```python
from build123d import *

# Parameters (mm, degrees)
SKETCH2_R                      = 2
BOSS_EXTRUDE1_DEPTH            = 10
CUT_EXTRUDE2_DEPTH             = 31.479501308
CUT_EXTRUDE2_DEPTH_BACK        = 31.479501308
SKETCH4_W                      = 15
SKETCH4_H                      = 9.2
CUT_EXTRUDE1_REACH             = 37.057
SKETCH3_R                      = 4.5
FILLET3_R                      = 1.5
FILLET4_R                      = 2
CUT_EXTRUDE3_REACH             = 31.082
SKETCH5_R                      = 9
CUT_EXTRUDE3_DIRECTION_2_REACH = 31.082
CUT_EXTRUDE4_DEPTH             = 3


with BuildPart() as part:
    # Sketch2 → Boss-Extrude1 (new, symmetric)
    with BuildSketch(Plane(origin=(0, 0, 0), x_dir=(1, 0, 0), z_dir=(0, 1, 0))):
        Polygon((-10, -9), (0, -27), (10, -9), (10, 9), (-10, 9), align=None)
        with Locations(Location((0, -17, 0), (0, 0, 270))):
            Circle(SKETCH2_R, mode=Mode.SUBTRACT)
    extrude(amount=BOSS_EXTRUDE1_DEPTH, both=True)

    # Sketch4 → Cut-Extrude2 (cut, two sides: drawn at the far end of the back side and taken through both)
    with BuildSketch(Plane(origin=(0, 0, 0), x_dir=(0, 0, -1), z_dir=(1, 0, 0)).offset(-CUT_EXTRUDE2_DEPTH_BACK)):
        with Locations((-19.5, 0)):
            Rectangle(SKETCH4_W, SKETCH4_H)
    extrude(amount=CUT_EXTRUDE2_DEPTH + CUT_EXTRUDE2_DEPTH_BACK, mode=Mode.SUBTRACT)

    # Sketch3 → Cut-Extrude1 (cut, up to next)
    with BuildSketch(Plane(origin=(10, 0, 0), x_dir=(0, 0, -1), z_dir=(1, 0, 0)), mode=Mode.PRIVATE) as cut_extrude1_sk1:
        Circle(SKETCH3_R)
    cut_extrude1_tool1 = extrude(cut_extrude1_sk1.sketch, amount=-CUT_EXTRUDE1_REACH, mode=Mode.PRIVATE) & part.part
    add(cut_extrude1_tool1.solids().sort_by_distance((10, 0, 0))[0], mode=Mode.SUBTRACT)

    # Fillet3
    fillet3_edges = [part.edges().sort_by_distance(p)[0] for p in [
        (0, 7.3, 27),
        (0, -7.3, 27),
    ]]
    fillet(fillet3_edges, radius=FILLET3_R)

    # Fillet4
    fillet4_edges = [part.edges().sort_by_distance(p)[0] for p in [
        (10, 0, 9),
        (-10, 0, 9),
        (-10, 0, -9),
        (10, 0, -9),
    ]]
    fillet(fillet4_edges, radius=FILLET4_R)

    # Cut-Extrude3: up to this face of the body (flat: up to its plane)
    cut_extrude3_end = Plane(part.part.faces().sort_by_distance((-4.635280123, -4.6, 18.215996288))[0])
    # Sketch5 → Cut-Extrude3 (cut, up to the picked face)
    with BuildSketch(Plane(origin=(0, 0, 0), x_dir=(1, 0, 0), z_dir=(0, 1, 0)), mode=Mode.PRIVATE) as cut_extrude3_sk1:
        with Locations((0, -17)):
            Circle(SKETCH5_R)
    cut_extrude3_tool1 = split(extrude(cut_extrude3_sk1.sketch, amount=-CUT_EXTRUDE3_REACH, mode=Mode.PRIVATE), bisect_by=cut_extrude3_end, keep=Keep.BOTH, mode=Mode.PRIVATE)
    add(cut_extrude3_tool1.solids().sort_by(Axis((0, 0, 17), (0, -1, 0)))[0], mode=Mode.SUBTRACT)

    # Cut-Extrude3 direction 2: up to this face of the body (flat: up to its plane)
    cut_extrude3_direction_2_end = Plane(part.part.faces().sort_by_distance((-4.635280123, 4.6, 18.215996288))[0])
    # Sketch5 → Cut-Extrude3 direction 2 (cut, up to the picked face)
    with BuildSketch(Plane(origin=(0, 0, 0), x_dir=(1, 0, 0), z_dir=(0, 1, 0)), mode=Mode.PRIVATE) as cut_extrude3_direction_2_sk1:
        with Locations((0, -17)):
            Circle(SKETCH5_R)
    cut_extrude3_direction_2_tool1 = split(extrude(cut_extrude3_direction_2_sk1.sketch, amount=CUT_EXTRUDE3_DIRECTION_2_REACH, mode=Mode.PRIVATE), bisect_by=cut_extrude3_direction_2_end, keep=Keep.BOTH, mode=Mode.PRIVATE)
    add(cut_extrude3_direction_2_tool1.solids().sort_by(Axis((0, 0, 17), (0, 1, 0)))[0], mode=Mode.SUBTRACT)

    # Sketch8 → Cut-Extrude4 (cut)
    with BuildSketch(Plane.XZ.offset(10)):
        with BuildLine():
            Line((2.205478028, 13.66), (3.100370946, 15.21))
            Line((3.100370946, 15.21), (3.995263863, 16.76))
            ThreePointArc((3.995263863, 16.76), (4.059571669, 17), (3.995263863, 17.24))
            Line((3.995263863, 17.24), (3.100370946, 18.79))
            Line((3.100370946, 18.79), (2.205478028, 20.34))
            ThreePointArc((2.205478028, 20.34), (2.029785834, 20.515692194), (1.789785834, 20.58))
            Line((1.789785834, 20.58), (0, 20.58))
            Line((0, 20.58), (-1.789785834, 20.58))
            ThreePointArc((-1.789785834, 20.58), (-2.029785834, 20.515692194), (-2.205478028, 20.34))
            Line((-2.205478028, 20.34), (-3.100370946, 18.79))
            Line((-3.100370946, 18.79), (-3.995263863, 17.24))
            ThreePointArc((-3.995263863, 17.24), (-4.059571669, 17), (-3.995263863, 16.76))
            Line((-3.995263863, 16.76), (-3.100370946, 15.21))
            Line((-3.100370946, 15.21), (-2.205478028, 13.66))
            ThreePointArc((-2.205478028, 13.66), (-2.029785834, 13.484307806), (-1.789785834, 13.42))
            Line((-1.789785834, 13.42), (0, 13.42))
            Line((0, 13.42), (1.789785834, 13.42))
            ThreePointArc((1.789785834, 13.42), (2.029785834, 13.484307806), (2.205478028, 13.66))
        make_face()
    extrude(amount=-CUT_EXTRUDE4_DEPTH, mode=Mode.SUBTRACT)


solid = part.part
```
The model under review builds one solid part; all positions refer to its coordinate system, in mm. A direction names the side the tool comes from. Coordinates: 2 decimals unless noted, no trailing zeros. Write each loop counter-clockwise with the first axis right and the second up, starting at its lowest first coordinate (ties: lowest second). Pieces come first, ordered by that corner, then holes.
1) We need section A-A on x = 0. State the section outline as (y, z) points.
2) We need section C-C on z = 0. State the section outline as (x, y) points, then the cut area to 3 significant figures.
3) We need section B-B on y = 0. State the section outline as (x, z) points, then the cut area to 3 significant figures.
4) We need section D-D on y = 5.25. State the section outline as (x, z) points.
5) Clearance check with flat-ended pins moving along their axes: pin 1 Ø5 at (x, z) = (0, 17) entering from -Y; pin 2 Ø3 at (x, z) = (0, 17) entering from -Y; pin 3 Ø10 at (x, z) = (0, 16.5) entering from -Y; pin 4 Ø10 at (x, y) = (5.5, 7) entering from +Z. State where each tip first meets the part, or that it passes through.
6) To check wall thickness, follow probe 1 along Y at (x, z) = (-5, 0); probe 2 along Y at (x, z) = (-5.5, 13); probe 3 along Z at (x, y) = (0, -5.7). State the ranges of each line that lie inside material, in increasing order.
7) The part is to be moulded in two halves that separate along Z. For faces 1 (the face through (0, -9, 20.58)), 2 (the face through (-9.43, -0.14, -8.4)), 3 (the face through (0.14, 4.46, 0.59)), 4 (the face through (-0.02, -7.26, 25.41)), say which applies: pulls with the +Z half, pulls with the -Z half, needs draft (parallel to the pull), parting line crosses it, or undercut.
8) Machinability: for faces 5 (the face through (-2, -7, 16)), 6 (the face through (9.4, -0.14, -8.43)), 7 (the face through (2, -4.6, 15)), 8 (the face through (-8, 0, 12)), which of the approach directions +Z, -Z, +X, -X, +Y, -Y give a long, thin tool a straight path to every point of the face, cutting with its end or side? Answer none if there is none.
Answer list:
1. outline: (-10, -9) - (10, -9) - (10, 15) - (4.6, 15) - (4.6, 8) - (-4.6, 8) - (-4.6, 15) - (-7, 15) - (-7, 13.42) - (-10, 13.42) - close; (-10, 20.58) - (-7, 20.58) - (-7, 19) - (-4.6, 19) - (-4.6, 25.41) - (-10, 25.41) - close; (4.6, 19) - (10, 19) - (10, 25.41) - (4.6, 25.41) - close; hole circle Ø9 at (0, 0)
2. outline: (-10, -10) - (10, -10) - (10, -4.5) - (-10, -4.5) - close; (-10, 4.5) - (10, 4.5) - (10, 10) - (-10, 10) - close
2. area: 220 mm2
3. outline: (-10, -7) arc R2 ccw to (-8, -9) - (8, -9) arc R2 ccw to (10, -7) - (10, -4.5) - (-10, -4.5) - close; (-10, 4.5) - (10, 4.5) - (10, 8.48) arc R2 ccw to (9.75, 9.45) - (8.33, 12) - (7.48, 12) arc R9 cw to (-7.48, 12) - (-8.33, 12) - (-9.75, 9.45) arc R2 ccw to (-10, 8.48) - close
3. area: 191 mm2
4. outline: (-10, -7) arc R2 ccw to (-8, -9) - (8, -9) arc R2 ccw to (10, -7) - (10, 8.48) arc R2 ccw to (9.75, 9.45) - (1.31, 24.64) arc R1.5 ccw to (-1.31, 24.64) - (-9.75, 9.45) arc R2 ccw to (-10, 8.48) - close; hole circle Ø4 at (0, 17)
5. pin 1: stops at y = -7
5. pin 2: passes through
5. pin 3: stops at y = -10
5. pin 4: stops at z = 25.33
6. probe 1: y = -10 to -4.5, 4.5 to 10
6. probe 2: y = -10 to -4.6, 4.6 to 10
6. probe 3: z = -9 to 15, 19 to 25.41
7. face 1: undercut
7. face 2: pulls with the -Z half
7. face 3: undercut
7. face 4: pulls with the +Z half
8. face 5: -Y
8. face 6: -Z, +X, +Y, -Y
8. face 7: +Z
8. face 8: +Z, +X, -X
